```python
from build123d import *

# Parameters (mm, degrees)
F0_W     = 50.8
F0_H     = 50.8
F1_DEPTH = 88.9
F2_W     = 21.774474
F2_H     = 21.774474
F2_W_2   = 21.389768
F2_H_2   = 21.697533
F3_DEPTH = 79.375
F2_W_3   = 21.082
F4_DEPTH = 86.36
F5_W     = 0.692474
F5_H     = 21.697533
F6_DEPTH = 79.375


with BuildPart() as f1:
    # F0 (on Top) → F1 (new body)
    with BuildSketch(Plane.XY):
        Rectangle(F0_W, F0_H)
    extrude(amount=F1_DEPTH)

    # F2 (on face) → F3 (cut)
    with BuildSketch(Plane.XY.offset(88.9)):
        with Locations((-12.079832, -12.233618)):
            Rectangle(F2_W, F2_H)
        with Locations((12.272187, -12.233618)):
            Rectangle(F2_W_2, F2_H)
        with Locations((12.272187, 12.1184)):
            Rectangle(F2_W_2, F2_H_2)
    extrude(amount=-F3_DEPTH, mode=Mode.SUBTRACT)

    # F2 (on face) → F4 (cut)
    with BuildSketch(Plane.XY.offset(88.9)):
        with Locations((-12.426069, 12.1184)):
            Rectangle(F2_W_3, F2_H_2)
        with Locations((-12.079832, -12.233618)):
            Rectangle(F2_W, F2_H)
        with Locations((12.272187, -12.233618)):
            Rectangle(F2_W_2, F2_H)
        with Locations((12.272187, 12.1184)):
            Rectangle(F2_W_2, F2_H_2)
    extrude(amount=-F4_DEPTH, mode=Mode.SUBTRACT)

    # F5 (on face) → F6 (cut)
    with BuildSketch(Plane.XY.offset(88.9)):
        with Locations((-1.538832, 12.1184)):
            Rectangle(F5_W, F5_H)
    extrude(amount=-F6_DEPTH, mode=Mode.SUBTRACT)


solid = f1.part
```
Here's how the part is built. I have some questions about the finished solid (model axes, mm). A direction names the side the tool comes from. Coordinates: 2 decimals unless noted, no trailing zeros. Loops run counter-clockwise (first coordinate to the right, second up) from the corner with the lowest first, then second, coordinate; pieces in that order, holes last. Notation, with made-up numbers: (-33.75, 85.25) - (1.25, 85.25) arc R25 cw to (1.25, 103.25) - close; hole circle Ø11 at (48.25, 70). An arc over 180 degrees is marked (long way). Return JSON: item names as keys, results as strings. Group by question number.
Item 1: On a 3-axis mill with a long thin cutter (end or side, diameter ignored), from which of +Z, -Z, +X, -X, +Y, -Y can I reach the whole of each face in a straight line? I mean faces 1 (the face through (0, 25.4, 44)), 2 (the face through (1.577, -12, 46)). Say none if no direction works.
Item 2: Will this pin go through, and if not, where does the flat tip stop? P1, Ø6.5, axis at x = -7.5, y = 10, coming from the +Z side.
Item 3: I need wall thicknesses on line 1 (X direction, y = -4.5, z = 11); line 2 (Y direction, x = -17, z = 61); line 3 (Z direction, x = 5.5, y = -16). Which ranges of each line are inside material? Lowest first, please. Write a range as from..to.
Item 4: If we section it at D-D on y = 18.5: Write out the boundary of the cut face in (x, z) (3 decimals).
Item 5: If we section it at A-A on z = 27: Write out the boundary of the cut face in (x, y).
Item 6: If we section it at B-B on y = -8: Write out the boundary of the cut face in (x, z).
Item 7: We'd pull the mould along X, two halves only. Please class faces 3 (the face through (0, 0, 0)), 4 (the face through (12, 12, 2.54)), 5 (the face through (25.4, 0, 44)): +X half, -X half, draft (parallel to the pull), parting line (faces both ways), or undercut.
Item 8: If we section it at C-C on x = -16: Write out the boundary of the cut face in (y, z).
Calculated:
{
 "1": {"face 1": "+Z, -Z, +X, -X, +Y", "face 2": "+Z"},
 "2": {"P1": "stops at z = 2.54"},
 "3": {"line 1": "x = -25.4..-22.97, -1.19..1.58, 22.97..25.4", "line 2": "y = -25.4..-23.12, -1.35..1.27, 22.97..25.4", "line 3": "z = 0..2.54"},
 "4": {"outline": "(-25.4, 0) - (25.4, 0) - (25.4, 88.9) - (22.967, 88.9) - (22.967, 2.54) - (1.577, 2.54) - (1.577, 88.9) - (-1.193, 88.9) - (-1.193, 9.525) - (-1.885, 9.525) - (-1.885, 2.54) - (-22.967, 2.54) - (-22.967, 88.9) - (-25.4, 88.9) - close"},
 "5": {"outline": "(-25.4, -25.4) - (25.4, -25.4) - (25.4, 25.4) - (-25.4, 25.4) - close; hole (-22.97, -23.12) - (-1.19, -23.12) - (-1.19, -1.35) - (-22.97, -1.35) - close; hole (-22.97, 1.27) - (-1.19, 1.27) - (-1.19, 22.97) - (-22.97, 22.97) - close; hole (1.58, -23.12) - (22.97, -23.12) - (22.97, -1.35) - (1.58, -1.35) - close; hole (1.58, 1.27) - (22.97, 1.27) - (22.97, 22.97) - (1.58, 22.97) - close"},
 "6": {"outline": "(-25.4, 0) - (25.4, 0) - (25.4, 88.9) - (22.97, 88.9) - (22.97, 2.54) - (1.58, 2.54) - (1.58, 88.9) - (-1.19, 88.9) - (-1.19, 2.54) - (-22.97, 2.54) - (-22.97, 88.9) - (-25.4, 88.9) - close"},
 "7": {"face 3": "draft", "face 4": "undercut", "face 5": "+X half"},
 "8": {"outline": "(-25.4, 0) - (25.4, 0) - (25.4, 88.9) - (22.97, 88.9) - (22.97, 2.54) - (1.27, 2.54) - (1.27, 88.9) - (-1.35, 88.9) - (-1.35, 2.54) - (-23.12, 2.54) - (-23.12, 88.9) - (-25.4, 88.9) - close"}
}
